from build123d import *

# Parameters (mm, degrees)
ESTRUSIONE_ESTRUSIONE1_DEPTH = 7.5
ESTRUSIONE_ESTRUSIONE2_DEPTH = 4
TAGLIO_ESTRUSIONE1_DEPTH     = 198.380910943
TAGLIO_ESTRUSIONE2_DEPTH     = 198.380910943
RACCORDO1_R                  = 25
FORO_PER_VITE_M6_5_1_D       = 7.5
TAGLIO_ESTRUSIONE3_DEPTH     = 7.5
TAGLIO_ESTRUSIONE4_DEPTH     = 7.5


with BuildPart() as part:
    # Schizzo1 → Estrusione-Estrusione1 (new, symmetric)
    with BuildSketch(Plane.XY):
        with BuildLine():
            Line((14.5, 182.011383906), (14.5, -37.988616094))
            ThreePointArc((14.5, -37.988616094), (0, -52.488616094), (-14.5, -37.988616094))
            Line((-14.5, -37.988616094), (-14.5, 182.011383906))
            ThreePointArc((-14.5, 182.011383906), (0, 196.511383906), (14.5, 182.011383906))
        make_face()
    extrude(amount=ESTRUSIONE_ESTRUSIONE1_DEPTH, both=True)

    # Schizzo2 → Estrusione-Estrusione2 (add, symmetric)
    with BuildSketch(Plane.XY):
        with BuildLine():
            Line((13, -40.066616094), (13, -56.066616094))
            ThreePointArc((13, -56.066616094), (0, -69.066616094), (-13, -56.066616094))
            Line((-13, -56.066616094), (-13, -40.066616094))
            ThreePointArc((-13, -40.066616094), (0, -27.066616094), (13, -40.066616094))
        make_face()
    extrude(amount=ESTRUSIONE_ESTRUSIONE2_DEPTH, both=True)

    # Schizzo4 → Taglio-Estrusione1 (cut, through all)
    with BuildSketch(Plane.XY.offset(4)):
        with BuildLine():
            Line((5.29445937, -51.487456784), (14.5, -37.988616094))
            Line((14.5, -37.988616094), (21.494330869, -44.738036439))
            Line((21.494330869, -44.738036439), (5.386515672, -60.537124892))
            ThreePointArc((5.386515672, -60.537124892), (0.071202698, -63.066253954), (-5.29445937, -60.645775404))
            Line((-5.29445937, -60.645775404), (-28.596127717, -39.453615031))
            Line((-28.596127717, -39.453615031), (-14.5, -31.562211214))
            Line((-14.5, -31.562211214), (-3.845832517, -50.217721134))
            ThreePointArc((-3.845832517, -50.217721134), (0.963165144, -49.133196093), (5.29445937, -51.487456784))
        make_face()
    taglio_estrusione1 = extrude(amount=TAGLIO_ESTRUSIONE1_DEPTH, mode=Mode.SUBTRACT)

    # Specchia1: Taglio-Estrusione1 across plane
    add(taglio_estrusione1.mirror(Plane.XY), mode=Mode.SUBTRACT)

    # Schizzo5 → Taglio-Estrusione2 (cut, through all)
    with BuildSketch(Plane.XY.offset(4)):
        Polygon((-13, -44.411232383), (-13, -34.188720036), (-15.056335757, -30.588064032), (-15.056335757, -43.619366988), align=None)
        Polygon((13, -44.411232383), (13, -40.188189356), (17.407959402, -33.724436261), (17.407959402, -44.411232383), align=None)
    extrude(amount=-TAGLIO_ESTRUSIONE2_DEPTH, mode=Mode.SUBTRACT)

    # Raccordo1
    # the kernel refuses this fillet: 25 mm, written as the material it takes off along each edge
    with BuildSketch(Plane(origin=(-14.5, -31.562211214, -24.089497944), x_dir=(0.4959240379913526, -0.8683659070589721, 0), z_dir=(0, 0, 1))) as raccordo1_piece_1_section:
        with BuildLine():
            CenterArc((RACCORDO1_R * 0.26543196711, RACCORDO1_R), RACCORDO1_R, 240.269299078, 29.730700922)
            Line((-RACCORDO1_R * 0.230492070882, RACCORDO1_R * 0.131634092941), (0, 0))
            Line((0, 0), (RACCORDO1_R * 0.26543196711, 0))
        make_face()
    raccordo1_piece_1 = extrude(amount=48.178995889, mode=Mode.PRIVATE)
    raccordo1_piece_1 = split(raccordo1_piece_1, bisect_by=Plane(origin=(-13, -35.788331904, -14.044748972), z_dir=(1, 0, 0)), keep=Keep.TOP, mode=Mode.PRIVATE)
    raccordo1_piece_1 = split(raccordo1_piece_1, bisect_by=Plane(origin=(-12.28179921, -35.788331904, -4), z_dir=(0, 0, -1)), keep=Keep.TOP, mode=Mode.PRIVATE)
    add(raccordo1_piece_1, mode=Mode.SUBTRACT)
    with BuildSketch(Plane(origin=(-14.5, -31.562211214, -24.089497944), x_dir=(0.4959240379913526, -0.8683659070589721, 0), z_dir=(0, 0, 1))) as raccordo1_piece_2_section:
        with BuildLine():
            CenterArc((RACCORDO1_R * 0.26543196711, RACCORDO1_R), RACCORDO1_R, 240.269299078, 29.730700922)
            Line((-RACCORDO1_R * 0.230492070882, RACCORDO1_R * 0.131634092941), (0, 0))
            Line((0, 0), (RACCORDO1_R * 0.26543196711, 0))
        make_face()
    raccordo1_piece_2 = extrude(amount=48.178995889, mode=Mode.PRIVATE)
    raccordo1_piece_2 = split(raccordo1_piece_2, bisect_by=Plane(origin=(-13, -30.370530988, -14.044748972), z_dir=(-1, 0, 0)), keep=Keep.TOP, mode=Mode.PRIVATE)
    raccordo1_piece_2 = split(raccordo1_piece_2, bisect_by=Plane(origin=(-14.266276842, -30.370530988, -4), z_dir=(0, 0, -1)), keep=Keep.TOP, mode=Mode.PRIVATE)
    add(raccordo1_piece_2, mode=Mode.SUBTRACT)
    with BuildSketch(Plane(origin=(-14.5, -31.562211214, -24.089497944), x_dir=(0.4959240379913526, -0.8683659070589721, 0), z_dir=(0, 0, 1))) as raccordo1_piece_3_section:
        with BuildLine():
            CenterArc((RACCORDO1_R * 0.26543196711, RACCORDO1_R), RACCORDO1_R, 240.269299078, 29.730700922)
            Line((-RACCORDO1_R * 0.230492070882, RACCORDO1_R * 0.131634092941), (0, 0))
            Line((0, 0), (RACCORDO1_R * 0.26543196711, 0))
        make_face()
    raccordo1_piece_3 = extrude(amount=48.178995889, mode=Mode.PRIVATE)
    raccordo1_piece_3 = split(raccordo1_piece_3, bisect_by=Plane(origin=(-14.266276842, -30.370530988, 4), z_dir=(0, 0, -1)), keep=Keep.TOP, mode=Mode.PRIVATE)
    raccordo1_piece_3 = split(raccordo1_piece_3, bisect_by=Plane(origin=(-13, -30.370530988, 0), z_dir=(-1, 0, 0)), keep=Keep.TOP, mode=Mode.PRIVATE)
    raccordo1_piece_3 = split(raccordo1_piece_3, bisect_by=Plane(origin=(-14.266276842, -30.370530988, -4), z_dir=(0, 0, 1)), keep=Keep.TOP, mode=Mode.PRIVATE)
    add(raccordo1_piece_3, mode=Mode.SUBTRACT)
    with BuildSketch(Plane(origin=(-14.5, -31.562211214, -24.089497944), x_dir=(0.4959240379913526, -0.8683659070589721, 0), z_dir=(0, 0, 1))) as raccordo1_piece_4_section:
        with BuildLine():
            CenterArc((RACCORDO1_R * 0.26543196711, RACCORDO1_R), RACCORDO1_R, 240.269299078, 29.730700922)
            Line((-RACCORDO1_R * 0.230492070882, RACCORDO1_R * 0.131634092941), (0, 0))
            Line((0, 0), (RACCORDO1_R * 0.26543196711, 0))
        make_face()
    raccordo1_piece_4 = extrude(amount=48.178995889, mode=Mode.PRIVATE)
    raccordo1_piece_4 = split(raccordo1_piece_4, bisect_by=Plane(origin=(-12.28179921, -35.788331904, 4), z_dir=(0, 0, 1)), keep=Keep.TOP, mode=Mode.PRIVATE)
    raccordo1_piece_4 = split(raccordo1_piece_4, bisect_by=Plane(origin=(-13, -35.788331904, 14.044748972), z_dir=(1, 0, 0)), keep=Keep.TOP, mode=Mode.PRIVATE)
    add(raccordo1_piece_4, mode=Mode.SUBTRACT)
    with BuildSketch(Plane(origin=(-14.5, -31.562211214, -24.089497944), x_dir=(0.4959240379913526, -0.8683659070589721, 0), z_dir=(0, 0, 1))) as raccordo1_piece_5_section:
        with BuildLine():
            CenterArc((RACCORDO1_R * 0.26543196711, RACCORDO1_R), RACCORDO1_R, 240.269299078, 29.730700922)
            Line((-RACCORDO1_R * 0.230492070882, RACCORDO1_R * 0.131634092941), (0, 0))
            Line((0, 0), (RACCORDO1_R * 0.26543196711, 0))
        make_face()
    raccordo1_piece_5 = extrude(amount=48.178995889, mode=Mode.PRIVATE)
    raccordo1_piece_5 = split(raccordo1_piece_5, bisect_by=Plane(origin=(-14.266276842, -30.370530988, 4), z_dir=(0, 0, 1)), keep=Keep.TOP, mode=Mode.PRIVATE)
    raccordo1_piece_5 = split(raccordo1_piece_5, bisect_by=Plane(origin=(-13, -30.370530988, 14.044748972), z_dir=(-1, 0, 0)), keep=Keep.TOP, mode=Mode.PRIVATE)
    add(raccordo1_piece_5, mode=Mode.SUBTRACT)
    with BuildSketch(Plane(origin=(14.5, -37.988616094, 26.782481556), x_dir=(0, 1, 0), z_dir=(0, 0, -1))) as raccordo1_piece_6_section:
        with BuildLine():
            CenterArc((RACCORDO1_R * 0.308519704891, -RACCORDO1_R), RACCORDO1_R, 90, 34.292050498)
            Line((-RACCORDO1_R * 0.254891721625, -RACCORDO1_R * 0.173823527041), (0, 0))
            Line((0, 0), (RACCORDO1_R * 0.308519704891, 0))
        make_face()
    raccordo1_piece_6 = extrude(amount=53.564963111, mode=Mode.PRIVATE)
    raccordo1_piece_6 = split(raccordo1_piece_6, bisect_by=Plane(origin=(14.242102238, -36.251699178, 4), z_dir=(0, 0, 1)), keep=Keep.TOP, mode=Mode.PRIVATE)
    raccordo1_piece_6 = split(raccordo1_piece_6, bisect_by=Plane(origin=(13, -36.251699178, 15.391240778), z_dir=(1, 0, 0)), keep=Keep.TOP, mode=Mode.PRIVATE)
    add(raccordo1_piece_6, mode=Mode.SUBTRACT)
    with BuildSketch(Plane(origin=(14.5, -37.988616094, 26.782481556), x_dir=(0, 1, 0), z_dir=(0, 0, -1))) as raccordo1_piece_7_section:
        with BuildLine():
            CenterArc((RACCORDO1_R * 0.308519704891, -RACCORDO1_R), RACCORDO1_R, 90, 34.292050498)
            Line((-RACCORDO1_R * 0.254891721625, -RACCORDO1_R * 0.173823527041), (0, 0))
            Line((0, 0), (RACCORDO1_R * 0.308519704891, 0))
        make_face()
    raccordo1_piece_7 = extrude(amount=53.564963111, mode=Mode.PRIVATE)
    raccordo1_piece_7 = split(raccordo1_piece_7, bisect_by=Plane(origin=(11.895384145, -41.966992208, 4), z_dir=(0, 0, 1)), keep=Keep.TOP, mode=Mode.PRIVATE)
    raccordo1_piece_7 = split(raccordo1_piece_7, bisect_by=Plane(origin=(13, -41.966992208, 15.391240778), z_dir=(-1, 0, 0)), keep=Keep.TOP, mode=Mode.PRIVATE)
    add(raccordo1_piece_7, mode=Mode.SUBTRACT)
    with BuildSketch(Plane(origin=(14.5, -37.988616094, 26.782481556), x_dir=(0, 1, 0), z_dir=(0, 0, -1))) as raccordo1_piece_8_section:
        with BuildLine():
            CenterArc((RACCORDO1_R * 0.308519704891, -RACCORDO1_R), RACCORDO1_R, 90, 34.292050498)
            Line((-RACCORDO1_R * 0.254891721625, -RACCORDO1_R * 0.173823527041), (0, 0))
            Line((0, 0), (RACCORDO1_R * 0.308519704891, 0))
        make_face()
    raccordo1_piece_8 = extrude(amount=53.564963111, mode=Mode.PRIVATE)
    raccordo1_piece_8 = split(raccordo1_piece_8, bisect_by=Plane(origin=(14.242102238, -36.251699178, 4), z_dir=(0, 0, -1)), keep=Keep.TOP, mode=Mode.PRIVATE)
    raccordo1_piece_8 = split(raccordo1_piece_8, bisect_by=Plane(origin=(14.242102238, -36.251699178, -4), z_dir=(0, 0, 1)), keep=Keep.TOP, mode=Mode.PRIVATE)
    raccordo1_piece_8 = split(raccordo1_piece_8, bisect_by=Plane(origin=(13, -36.251699178, 0), z_dir=(1, 0, 0)), keep=Keep.TOP, mode=Mode.PRIVATE)
    add(raccordo1_piece_8, mode=Mode.SUBTRACT)
    with BuildSketch(Plane(origin=(14.5, -37.988616094, 26.782481556), x_dir=(0, 1, 0), z_dir=(0, 0, -1))) as raccordo1_piece_9_section:
        with BuildLine():
            CenterArc((RACCORDO1_R * 0.308519704891, -RACCORDO1_R), RACCORDO1_R, 90, 34.292050498)
            Line((-RACCORDO1_R * 0.254891721625, -RACCORDO1_R * 0.173823527041), (0, 0))
            Line((0, 0), (RACCORDO1_R * 0.308519704891, 0))
        make_face()
    raccordo1_piece_9 = extrude(amount=53.564963111, mode=Mode.PRIVATE)
    raccordo1_piece_9 = split(raccordo1_piece_9, bisect_by=Plane(origin=(14.242102238, -36.251699178, -4), z_dir=(0, 0, -1)), keep=Keep.TOP, mode=Mode.PRIVATE)
    raccordo1_piece_9 = split(raccordo1_piece_9, bisect_by=Plane(origin=(13, -36.251699178, -15.391240778), z_dir=(1, 0, 0)), keep=Keep.TOP, mode=Mode.PRIVATE)
    add(raccordo1_piece_9, mode=Mode.SUBTRACT)
    with BuildSketch(Plane(origin=(14.5, -37.988616094, 26.782481556), x_dir=(0, 1, 0), z_dir=(0, 0, -1))) as raccordo1_piece_10_section:
        with BuildLine():
            CenterArc((RACCORDO1_R * 0.308519704891, -RACCORDO1_R), RACCORDO1_R, 90, 34.292050498)
            Line((-RACCORDO1_R * 0.254891721625, -RACCORDO1_R * 0.173823527041), (0, 0))
            Line((0, 0), (RACCORDO1_R * 0.308519704891, 0))
        make_face()
    raccordo1_piece_10 = extrude(amount=53.564963111, mode=Mode.PRIVATE)
    raccordo1_piece_10 = split(raccordo1_piece_10, bisect_by=Plane(origin=(11.895384145, -41.966992208, -4), z_dir=(0, 0, -1)), keep=Keep.TOP, mode=Mode.PRIVATE)
    raccordo1_piece_10 = split(raccordo1_piece_10, bisect_by=Plane(origin=(13, -41.966992208, -15.391240778), z_dir=(-1, 0, 0)), keep=Keep.TOP, mode=Mode.PRIVATE)
    add(raccordo1_piece_10, mode=Mode.SUBTRACT)

    # Foro per Vite M6.5-1 (through all)
    with Locations(Plane(origin=(0, -56.066616094, 4), x_dir=(1, 0, 0), z_dir=(0, 0, 1))):
        with Locations((0, 0)):
            Hole(FORO_PER_VITE_M6_5_1_D / 2)

    # Schizzo8 → Taglio-Estrusione3 (cut, symmetric)
    with BuildSketch(Plane.XY):
        with BuildLine():
            Line((9, 182.011383906), (9, -27.988616094))
            ThreePointArc((9, -27.988616094), (0, -36.988616094), (-9, -27.988616094))
            Line((-9, -27.988616094), (-9, 182.011383906))
            ThreePointArc((-9, 182.011383906), (0, 191.011383906), (9, 182.011383906))
        make_face()
    extrude(amount=TAGLIO_ESTRUSIONE3_DEPTH, both=True, mode=Mode.SUBTRACT)

    # Schizzo9 → Taglio-Estrusione4 (cut)
    with BuildSketch(Plane.XY.offset(7.5)):
        with BuildLine():
            Line((-9, 182.011383906), (-9, 202.011383906))
            ThreePointArc((-9, 202.011383906), (0, 211.011383906), (9, 202.011383906))
            Line((9, 202.011383906), (9, 182.011383906))
            ThreePointArc((9, 182.011383906), (0, 173.011383906), (-9, 182.011383906))
        make_face()
    extrude(amount=-TAGLIO_ESTRUSIONE4_DEPTH, mode=Mode.SUBTRACT)


solid = part.part
CAD build for the part. Positions are in the model's coordinates, mm. A direction names the side the tool comes from. Coordinates: 2 decimals unless noted, no trailing zeros. Loops run counter-clockwise (first coordinate to the right, second up) from the corner with the lowest first, then second, coordinate; pieces in that order, holes last. Notation, with made-up numbers: (43.25, 24.25) -> (58.25, 24.25) arc R19 ccw to (58.25, 58.25) -> close; hole circle Ø8 at (82.5, 28). An arc over 180 degrees is marked (long way). One line per item, written item: value.
1. Which spindle directions (+Z, -Z, +X, -X, +Y, -Y) get a long thin tool onto all of the face, cutting with end or side? Do faces 5 (the face through (0, 193, 0)), 6 (the face through (-7.58, -43.68, 5.73)), 7 (the face through (-3, -59, -4)). Say none if no direction does.
Answers:
face 5: +Z, +Y
face 6: +Z, -X, -Y
face 7: -Z, -Y
2. Slice it at A-A on x = 0. Write the cut outline in (y, z).
Answers:
outline: (-69.07, -4) -> (-59.82, -4) -> (-59.82, 4) -> (-69.07, 4) -> close; (-52.32, -4) -> (-49.07, -4) -> (-49.07, -7.5) -> (-36.99, -7.5) -> (-36.99, 7.5) -> (-49.07, 7.5) -> (-49.07, 4) -> (-52.32, 4) -> close; (191.01, -7.5) -> (196.51, -7.5) -> (196.51, 0) -> (191.01, 0) -> close
3. Drill centre lines: line 1 (X direction, y = 19, z = 5); line 2 (Y direction, x = 0, z = 2.75); line 3 (Y direction, x = 1, z = -6.5). Where is each one in solid material? Low to high. Write a range as [from, to].
Answers:
line 1: x = [-14.5, -9], [9, 14.5]
line 2: y = [-69.07, -59.82], [-52.32, -36.99]
line 3: y = [-49.14, -36.93], [190.96, 196.48]
4. Slice it at B-B on y = 45.5. Write the cut outline in (x, z), and give its area (3 significant figures).
Answers:
outline: (-14.5, -7.5) -> (-9, -7.5) -> (-9, 7.5) -> (-14.5, 7.5) -> close; (9, -7.5) -> (14.5, -7.5) -> (14.5, 7.5) -> (9, 7.5) -> close
area: 165 mm^2
5. Pull direction X, two halves, no side cores. Call faces 1 (the face through (0.81, -59.73, -0.06)), 2 (the face through (7.69, -47.974, 5.726)), 3 (the face through (-14.01, -29.85, -0.11)), 4 (the face through (9, 84, 0)): pulls with the +X half, pulls with the -X half, needs draft (parallel to the pull), parting line crosses it, or undercut.
Answers:
face 1: undercut
face 2: pulls with the +X half
face 3: pulls with the -X half
face 4: undercut
6. Flat gauge pins, fed straight in: P1, Ø9, axis at y = -49.5, z = 0.5, coming from the +X side; P2, Ø4, axis at x = 3, z = 0.5, coming from the +Y side; P3, Ø4.5, axis at x = 0, y = -56.07, coming from the -Z side; P4, Ø9, axis at y = -48.5, z = -0.5, coming from the -X side. Where does each tip first touch, or does it go through?
Answers:
P1: stops at x = 13
P2: stops at y = 196.47
P3: passes through
P4: stops at x = -13
